Autodesk Inventor part; units mm, degrees
ref_plane "YZ Plane" through (0, 0, 0) normal (1, 0, 0) x (0, 1, 0)
ref_plane "XZ Plane" through (0, 0, 0) normal (0, 1, 0) x (-1, 0, 0)
ref_plane "XY Plane" through (0, 0, 0) normal (0, 0, 1) x (1, 0, 0)
sketch "스케치1" plane through (0, 0, 0) normal (0, 0, 1) x (1, 0, 0)
  line L0 (0, 0) -> (80, 0)
  line L1 (80, 0) -> (80, 36)
  line L2 (80, 36) -> (0, 36)
  line L3 (0, 36) -> (0, 0)
  dimension "d0" = 80
  dimension "d1" = 36
extrude "돌출1" add sketch "스케치1" along normal blind 1.5
sketch "스케치2" plane through (0, 0, 1.5) normal (0, 0, 1) x (1, 0, 0)
  line L0 (80, 36) -> (0, 36)
  line L1 (0, 36) -> (0, 0)
  line L2 (4.5, 30.5) -> (76, 30.5)
  line L3 (76, 30.5) -> (76, 3.5)
  line L4 (76, 3.5) -> (4.5, 3.5)
  line L5 (4.5, 3.5) -> (4.5, 30.5)
  dimension "d4" = 71.5
  dimension "d5" = 27
  dimension "d6" = 5.5
  dimension "d7" = 4.5
extrude "돌출2" add sketch "스케치2" along normal blind 8
sketch "스케치3" plane through (0, 0, 1.5) normal (0, 0, 1) x (1, 0, 0)
  line L0 (76, 30.5) -> (76, 3.5)
  line L1 (76, 24.5) -> (76, 9.5)
  line L2 (80, 20) -> (80, 14)
  line L3 (76, 24.5) -> (80, 20)
  line L4 (80, 14) -> (76, 9.5)
  point P0 (80, 36)
  point P1 (76, 17)
  point P2 (80, 17)
  point P3 (76, 17)
  dimension "d10" = 15
  dimension "d11" = 6
extrude "돌출3" add sketch "스케치3" along normal blind 2.5
sketch "스케치5" plane through (0, 0, 9.5) normal (0, 0, 1) x (1, 0, 0)
  line L0 (76, 30.5) -> (4.5, 30.5)
  line L1 (4.5, 30.5) -> (4.5, 3.5)
  line L2 (72.25, 23.75) -> (8.25, 23.75)
  line L3 (8.25, 23.75) -> (8.25, 10.25)
  line L4 (8.25, 10.25) -> (72.25, 10.25)
  line L5 (72.25, 10.25) -> (72.25, 23.75)
  line L6 (72.25, 23.75) -> (8.25, 10.25) construction
  line L7 (8.25, 23.75) -> (72.25, 10.25) construction
  point P0 (0, 0)
  point P1 (40.25, 17)
  point P2 (40.25, 17)
  point P3 (4.5, 17)
  point P4 (40.25, 17)
  point P5 (40.25, 30.5)
  dimension "d15" = 64
  dimension "d16" = 13.5
extrude "돌출4" cut sketch "스케치5" against normal blind 0.8
sketch "스케치6" plane through (0, 0, 1.5) normal (0, 0, 1) x (1, 0, 0)
  line L0 (80, 20) -> (80, 36)
  line L1 (80, 36) -> (0, 36)
  line L2 (0, 36) -> (0, 0)
  line L3 (0, 0) -> (80, 0)
  circle A0 centre (2.5, 33.5) radius 1.5
  circle A1 centre (77.5, 33.5) radius 1.5
  circle A2 centre (77.5, 2.5) radius 1.5
  circle A3 centre (2.5, 2.5) radius 1.5
  dimension "d19" = 80
  dimension "d20" = 3
  dimension "d21" = 3
  dimension "d22" = 3
  dimension "d23" = 3
  dimension "d24" = 1
  dimension "d25" = 1
  dimension "d26" = 1
  dimension "d27" = 1
extrude "돌출5" cut sketch "스케치6" against normal through all
sketch "스케치7" plane through (0, 0, 9.5) normal (0, 0, 1) x (1, 0, 0)
  line L0 (8.25, 10.25) -> (8.25, 23.75)
  line L1 (8.25, 23.75) -> (72.25, 23.75)
  line L2 (72.25, 23.75) -> (72.25, 10.25)
  line L3 (72.25, 10.25) -> (8.25, 10.25)
  line L4 (76, 30.5) -> (4.5, 30.5)
  line L5 (4.5, 30.5) -> (4.5, 3.5)
  line L6 (4.5, 3.5) -> (76, 3.5)
  line L7 (76, 3.5) -> (76, 30.5)
  circle A0 centre (77.5, 2.5) radius 1.5
  circle A1 centre (2.5, 33.5) radius 1.5
  circle A2 centre (77.5, 33.5) radius 1.5
  circle A3 centre (2.5, 2.5) radius 1.5
  line L8 (76, 24.5) -> (80, 20)
  line L9 (80, 20) -> (80, 36)
  line L10 (80, 36) -> (0, 36)
  line L11 (0, 36) -> (0, 0)
  line L12 (0, 0) -> (80, 0)
  line L13 (80, 0) -> (80, 14)
  line L14 (80, 14) -> (76, 9.5)
  line L15 (76, 9.5) -> (76, 3.5)
  line L16 (76, 3.5) -> (4.5, 3.5)
  line L17 (4.5, 3.5) -> (4.5, 30.5)
  line L18 (4.5, 30.5) -> (76, 30.5)
  line L19 (76, 30.5) -> (76, 24.5)
  line L20 (2.5, 33.5) -> (77.5, 33.5)
  line L21 (77.5, 33.5) -> (77.5, 2.5)
  line L22 (77.5, 2.5) -> (2.5, 2.5)
  line L23 (2.5, 2.5) -> (2.5, 33.5)
  line L24 (40, 33.5) -> (40, -15.5556)
  line L25 (2.5, 18) -> (93.9243, 18)
  line L26 (8.25, 17) -> (83.8017, 17) construction
  line L27 (40.25, 23.75) -> (40.25, -12.7239) construction
  line L28 (40, 18) -> (40.25, 18)
  line L29 (40.25, 18) -> (40.25, 17)
  dimension "d30" = 80
  dimension "d31" = 36
  dimension "d32" = 75
  dimension "d33" = 31
  dimension "d34" = 71.5
  dimension "d35" = 27
  dimension "d36" = 1
  dimension "d37" = 0.25
properties part number "1806LCD"
Build history of the part. All positions in model axes, mm. A direction names the side the tool comes from. Coordinates: 2 decimals unless noted, no trailing zeros. Order: outer loops, then holes, each group sorted by start corner. A loop starts at its lowest first (then second) coordinate and runs counter-clockwise, first axis right, second up. Notation, with made-up numbers: M -13,42.25 L 32,42.25 A29 cw 32,66.25 Z; hole C 51,72.5 d11. An arc over 180 degrees is marked long. One line per question, with ' | ' between items. Start each with the question number.
Q1. Saw through at A-A (x = 2.5). List the corners of the cut face in (y, z), then the cut area to 3 significant figures.
Q2. Probe L1, parallel to Y at x = 77.5, z = 1.15; L2, parallel to Y at x = 63.5, z = 8.75; L3, parallel to X at y = 10.5, z = 9. List the from-to ranges inside material, lowest first. Write a range as from..to.
Q3. Flat gauge pins, fed straight in: pin 1 Ø1 at (y, z) = (25.5, 1) entering from -X; pin 2 Ø2.5 at (y, z) = (18, 7) entering from -X; pin 3 Ø4 at (x, z) = (24, 5.5) entering from -Y; pin 4 Ø1.5 at (x, y) = (18, 21) entering from +Z. Where does each tip first touch, or does it go through?
Q4. Saw through at C-C (x = 70). List the corners of the cut face in (y, z).
Q5. Saw through at D-D (z = 3). List the corners of the cut face in (x, y).
Q6. Saw through at B-B (y = 33.5). List the corners of the cut face in (x, z), then the cut area to 3 significant figures.
Q7. 3-axis set-ups, long thin cutter, end or side, ignore diameter. For faces 4 (the face through (78.028, 11.781, 2.732)), 5 (the face through (40, 30.5, 5)), 6 (the face through (40, 17, 8.7)): which of +Z, -Z, +X, -X, +Y, -Y reach the whole face in a straight line?
Q8. Two-plate mould, pull along X, no slides. Class faces 1 (the face through (77.972, 22.281, 2.732)), 2 (the face through (78.93, 2.95, 0.76)), 3 (the face through (40, 8, 9.5)): +X half, -X half, draft (parallel to the pull), parting line (faces both ways), or undercut.
Check values:
1) outline: M 0,0 L 1,0 L 1,1.5 L 0,1.5 Z; M 4,0 L 32,0 L 32,1.5 L 4,1.5 Z; M 35,0 L 36,0 L 36,1.5 L 35,1.5 Z | area: 45.0 mm2
2) L1: y = 0..1, 4..32, 35..36 | L2: y = 3.5..10.25, 23.75..30.5 | L3: x = 4.5..8.25, 72.25..76
3) pin 1: stops at x = 0 | pin 2: stops at x = 4.5 | pin 3: stops at y = 3.5 | pin 4: stops at z = 8.7
4) outline: M 0,0 L 36,0 L 36,1.5 L 30.5,1.5 L 30.5,9.5 L 23.75,9.5 L 23.75,8.7 L 10.25,8.7 L 10.25,9.5 L 3.5,9.5 L 3.5,1.5 L 0,1.5 Z
5) outline: M 4.5,3.5 L 76,3.5 L 76,9.5 L 80,14 L 80,20 L 76,24.5 L 76,30.5 L 4.5,30.5 Z
6) outline: M 0,0 L 1,0 L 1,1.5 L 0,1.5 Z; M 4,0 L 76,0 L 76,1.5 L 4,1.5 Z; M 79,0 L 80,0 L 80,1.5 L 79,1.5 Z | area: 111 mm2
7) face 4: +Z, +X, -Y | face 5: +Z, +X, -X, +Y | face 6: +Z
8) face 1: +X half | face 2: undercut | face 3: draft
